```python
from build123d import *

# Parameters (mm, degrees)
ESQUISSE1_R             = 45
BASE_EXTRUSION_DEPTH    = 100
ESQUISSE2_R             = 30
ENL_V_MAT_EXTRU_1_DEPTH = 100
ESQUISSE3_R             = 3
ENL_V_MAT_EXTRU_2_DEPTH = 30
CONG_1_R                = 2


with BuildPart() as part:
    # Esquisse1 → Base-Extrusion (new body)
    with BuildSketch(Plane.XY):
        Circle(ESQUISSE1_R)
    extrude(amount=BASE_EXTRUSION_DEPTH)

    # Esquisse2 → Enlèv. mat.-Extru.1 (cut)
    with BuildSketch(Plane.XY.offset(100)):
        Circle(ESQUISSE2_R)
    extrude(amount=-ENL_V_MAT_EXTRU_1_DEPTH, mode=Mode.SUBTRACT)

    # Esquisse3 → Enlèv. mat.-Extru.2 (cut)
    with BuildSketch(Plane.XY.offset(100)):
        with Locations((37.5, 0)):
            Circle(ESQUISSE3_R)
    extrude(amount=-ENL_V_MAT_EXTRU_2_DEPTH, mode=Mode.SUBTRACT)

    # Congé1
    cong_1_edges = [part.edges().sort_by_distance(p)[0] for p in [
        (-45, 0, 0),
    ]]
    fillet(cong_1_edges, radius=CONG_1_R)


solid = part.part
```
Check sheet for the modelled part. Datum: model origin and axes. Units: mm. A direction names the side the tool comes from. Give positions to 0.01 mm unless a question says otherwise; leave off trailing zeros. Order: outer loops, then holes, each group sorted by start corner. A loop starts at its lowest first (then second) coordinate and runs counter-clockwise, first axis right, second up. Notation, with made-up numbers: M -32.75,29.5 L 10.25,29.5 A21 cw 10.25,51.5 Z; hole C 42.25,5.25 d6. An arc over 180 degrees is marked long. Answer in a Markdown table with one row per item. Add a question column.
Q1. Thickness scan on L1, parallel to Y at x = -0.5, z = 50; L2, parallel to Y at x = -12.5, z = 70; L3, parallel to X at y = -23, z = 76.5. Record the ranges inside material, lowest first.
Q2. Sectioned sample at A-A, the plane x = 0. Record the boundary of the cut face in (y, z), and give its area (3 significant figures).
Q3. Sectioned sample at C-C, the plane z = 64. Record the boundary of the cut face in (x, y), and give its area (3 significant figures).
Q4. Sectioned sample at D-D, the plane z = 83.5. Record the boundary of the cut face in (x, y), and give its area (3 significant figures).
Q5. Release check for a two-part mould opening along Y. For faces 3 (the flat face through (9, -29, 100)), 4 (the flat face through (37, 0, 70)), 5 (the cylindrical face through (20.765, -39.923, 50.314)) record: released by +Y, released by -Y, zero draft, split by the parting line, or undercut.
Q6. Gauge pin test, flat ends, axial feed: pin 1 Ø2 at (y, z) = (-14.5, 32.5) entering from +X; pin 2 Ø1.5 at (x, z) = (18.5, 18) entering from -Y; pin 3 Ø1.5 at (x, z) = (17.5, 82) entering from -Y. Record the tip position at first contact, or that the pin passes through.
Q7. Sectioned sample at B-B, the plane y = 0. Record the boundary of the cut face in (x, z), and give its area (3 significant figures).
Q8. Access from +Z, -Z, +X, -X, +Y, -Y to the whole of each face (thin tool, end or side, straight path). Record for faces 1 (the cylindrical face through (-29.97, 1.32, 50.7)), 2 (the cylindrical face through (34.5, 0.1, 85.2)).
Verdict:
| question | item | result |
|---|---|---|
| 1 | L1 | -45 to -30, 30 to 45 |
| 1 | L2 | -43.23 to -27.27, 27.27 to 43.23 |
| 1 | L3 | -38.68 to -19.26, 19.26 to 38.68 |
| 2 | outline | M -45,2 A2 ccw -43,0 L -30,0 L -30,100 L -45,100 Z; M 30,0 L 43,0 A2 ccw 45,2 L 45,100 L 30,100 Z |
| 2 | area | 3,000 mm² |
| 3 | outline | C 0,0 d90; hole C 0,0 d60 |
| 3 | area | 3,530 mm² |
| 4 | outline | C 0,0 d90; hole C 0,0 d60; hole C 37.5,0 d6 |
| 4 | area | 3,510 mm² |
| 5 | face 3 | zero draft |
| 5 | face 4 | undercut |
| 5 | face 5 | split by the parting line |
| 6 | pin 1 | x = 42.93 |
| 6 | pin 2 | y = -41.35 |
| 6 | pin 3 | y = -41.77 |
| 7 | outline | M -45,2 A2 ccw -43,0 L -30,0 L -30,100 L -45,100 Z; M 30,0 L 43,0 A2 ccw 45,2 L 45,100 L 40.5,100 L 40.5,70 L 34.5,70 L 34.5,100 L 30,100 Z |
| 7 | area | 2,820 mm² |
| 8 | face 1 | +Z, -Z |
| 8 | face 2 | +Z |
